```python
from build123d import *
from build123d.topology import SkipClean

# Parameters (mm, degrees)
EXTRUDE_1_DEPTH      = 2
SKETCH_3_W           = 2
SKETCH_3_H           = 2
EXTRUDE_3_DEPTH      = 4
SKETCH_4_W           = 1.3
SKETCH_4_H           = 2
EXTRUDE_4_DEPTH      = 6.5
SKETCH_5_W           = 2
SKETCH_5_H           = 11
EXTRUDE_5_DEPTH      = 2
CHAMFER_1_SIZE       = 0.5
SKETCH_6_R           = 1.5
CUT_EXTRUDE_1_DEPTH  = 2
EXTRUDE_6_DEPTH      = 2
EXTRUDE_6_DEPTH_BACK = 6
CUT_EXTRUDE_START    = -2
CUT_EXTRUDE_2_DEPTH  = 2


with BuildPart() as part:
    # 草图1 → 凸台-拉伸1 (new body)
    with BuildSketch(Plane(origin=(0, 0, 0), x_dir=(0, 0, -1), z_dir=(1, 0, 0))):
        Polygon((-5.5, -3), (5.5, -3), (5.5, 3), (3.4, 3), (3.4, 5), (1.4, 5), (1.4, 3), (-1.4, 3), (-1.4, 5), (-3.4, 5), (-3.4, 3), (-5.5, 3), align=None)
    extrude(amount=EXTRUDE_1_DEPTH)

    # 草图3 → 凸台-拉伸3 (add)
    with BuildSketch(Plane(origin=(2, 0, 0), x_dir=(0, 0, -1), z_dir=(1, 0, 0))):
        with Locations((-2.4, 4)):
            Rectangle(SKETCH_3_W, SKETCH_3_H)
        with Locations((2.4, 4)):
            Rectangle(SKETCH_3_W, SKETCH_3_H)
    extrude(amount=EXTRUDE_3_DEPTH)

    # 草图4 → 凸台-拉伸4 (add)
    with BuildSketch(Plane.XZ.offset(-3)):
        with Locations((5.35, 2.4)):
            Rectangle(SKETCH_4_W, SKETCH_4_H)
        with Locations((5.35, -2.4)):
            Rectangle(SKETCH_4_W, SKETCH_4_H)
    extrude(amount=EXTRUDE_4_DEPTH)

    # 草图5 → 凸台-拉伸5 (add)
    with BuildSketch(Plane.XZ.offset(3)):
        with Locations((1, 0)):
            Rectangle(SKETCH_5_W, SKETCH_5_H)
    extrude(amount=EXTRUDE_5_DEPTH)

    # 倒角1
    chamfer_1_edges = [part.edges().sort_by_distance(p)[0] for p in [
        (6, 5, -2.4),
        (6, 5, 2.4),
    ]]
    chamfer(chamfer_1_edges, length=CHAMFER_1_SIZE)

    # 草图6 → 切除-拉伸1 (cut)
    with BuildSketch(Plane.ZY):
        Circle(SKETCH_6_R)
    extrude(amount=-CUT_EXTRUDE_1_DEPTH, mode=Mode.SUBTRACT)

    # 草图2 → 凸台-拉伸6 (add, two sides: drawn at the far end of the back side and taken through both)
    with SkipClean():  # the faces are left unmerged after this step: merging them gives an invalid solid
        with BuildSketch(Plane.XZ.offset(3).offset(-EXTRUDE_6_DEPTH_BACK)):
            with BuildLine():
                Line((-2.3, 10.512451089), (-2.3, 9.464007706))
                ThreePointArc((-2.3, 9.464007706), (0.5, 0), (-2.3, -9.464007706))
                Line((-2.3, -9.464007706), (-2.3, -10.512451089))
                ThreePointArc((-2.3, -10.512451089), (-1.949751675, -10.989498714), (-1.389702257, -10.798205813))
                ThreePointArc((-1.389702257, -10.798205813), (2, 0), (-1.389702257, 10.798205813))
                ThreePointArc((-1.389702257, 10.798205813), (-1.949751675, 10.989498714), (-2.3, 10.512451089))
            make_face()
        extrude(amount=EXTRUDE_6_DEPTH + EXTRUDE_6_DEPTH_BACK)

    # 草图7 → 切除-拉伸2 (cut)
    with SkipClean():  # the faces are left unmerged after this step: merging them gives an invalid solid
        with BuildSketch(Plane(origin=(2, 0, 0), x_dir=(0, 0, -1), z_dir=(1, 0, 0)).offset(CUT_EXTRUDE_START)):
            with BuildLine():
                ThreePointArc((0, -1.5), (1.5, 0), (0, 1.5))
                ThreePointArc((0, 1.5), (-1.5, 0), (0, -1.5))
            make_face()
        extrude(amount=CUT_EXTRUDE_2_DEPTH, mode=Mode.SUBTRACT)


solid = part.part
```
Geometry: final body of the model. Coordinates: model frame, mm. A direction names the side the tool comes from. Coordinates: 2 decimals unless noted, no trailing zeros. Order: outer loops, then holes, each group sorted by start corner. A loop starts at its lowest first (then second) coordinate and runs counter-clockwise, first axis right, second up. Notation, with made-up numbers: (1.25, -18) -> (16.25, -18) arc R25 cw to (16.25, 4) -> close; hole circle Ø10 at (39.5, 61). An arc over 180 degrees is marked (long way). Answer in a Markdown table with one row per item.
Item 1: Section C-C on y = 2.25. Output: boundary loops of the cut face in (x, z).
Return value:
| item | result |
|---|---|
| outline | (-2.3, -10.51) arc R0.5 ccw to (-1.39, -10.8) arc R18.89 ccw to (1.18, -5.5) -> (2, -5.5) -> (2, 5.5) -> (1.18, 5.5) arc R18.89 ccw to (-1.39, 10.8) arc R0.5 ccw to (-2.3, 10.51) -> (-2.3, 9.46) arc R17.39 cw to (0, 4.14) -> (0, -4.14) arc R17.39 cw to (-2.3, -9.46) -> close; (4.7, -3.4) -> (6, -3.4) -> (6, -1.4) -> (4.7, -1.4) -> close; (4.7, 1.4) -> (6, 1.4) -> (6, 3.4) -> (4.7, 3.4) -> close |
Item 2: Contact query for flat-ended pins moving along their axis: P1, Ø0.6, axis at x = 2.5, z = -3, coming from the -Y side; P2, Ø2, axis at y = 2, z = 5.5, coming from the -X side; P3, Ø2, axis at x = 2, z = 7, coming from the -Y side; P4, Ø1.7, axis at x = 1.5, z = 0, coming from the +Y side. Output: stop coordinate, or through.
Return value:
| item | result |
|---|---|
| P1 | stops at y = 3 |
| P2 | stops at x = -0.76 |
| P3 | passes through |
| P4 | stops at y = 3 |
Item 3: Draft query along X for faces 5 (the cylindrical face through (0.086, -0.944, -8.287)), 6 (the flat face through (3, 3, -2)), 7 (the flat face through (-2.3, -1, -10)). Return one class per face: released by +X, released by -X, zero draft, split by the parting line, or undercut.
Return value:
| item | result |
|---|---|
| face 5 | released by +X |
| face 6 | undercut |
| face 7 | released by -X |
Item 4: Ray query, L1, parallel to Y at x = 0.45, z = 0; L2, parallel to X at y = 0.75, z = -2.5; L3, parallel to Z at x = 1.65, y = 0. Return the intervals inside material, ascending.
Return value:
| item | result |
|---|---|
| L1 | y = -5 to -1.5, 1.5 to 3 |
| L2 | x = 0 to 2, 4.7 to 6 |
| L3 | z = -5.5 to -1.5, 1.5 to 5.5 |
Item 5: Access query for faces 1 (the flat face through (5, 3, -3.4)), 2 (the cylindrical face through (-0.91, -0.94, -6.86)), 3 (the flat face through (4.7, 0, 2)), 4 (the flat face through (5, -3.5, 2)). Directions: +Z, -Z, +X, -X, +Y, -Y. A direction counts if a zero-diameter tool reaches every point of the face in a straight line with its end or side. Return the directions, or none.
Return value:
| item | result |
|---|---|
| face 1 | -Z, +X, +Y |
| face 2 | -X, +Y, -Y |
| face 3 | +Z, -Z, -Y |
| face 4 | +Z, -Z, +X, -Y |
Item 6: Section B-B on x = 4.25. Output: boundary loops of the cut face in (y, z).
Return value:
| item | result |
|---|---|
| outline | (3, -3.4) -> (5, -3.4) -> (5, -1.4) -> (3, -1.4) -> close; (3, 1.4) -> (5, 1.4) -> (5, 3.4) -> (3, 3.4) -> close |
Item 7: Section D-D on y = 0.75. Output: boundary loops of the cut face in (x, z), plus the area to 3 significant figures.
Return value:
| item | result |
|---|---|
| outline | (-2.3, -10.51) arc R0.5 ccw to (-1.39, -10.8) arc R18.89 ccw to (1.18, -5.5) -> (2, -5.5) -> (2, -1.3) -> (0, -1.3) -> (0, -4.14) arc R17.39 cw to (-2.3, -9.46) -> close; (-2.3, 9.46) arc R17.39 cw to (0, 4.14) -> (0, 1.3) -> (2, 1.3) -> (2, 5.5) -> (1.18, 5.5) arc R18.89 ccw to (-1.39, 10.8) arc R0.5 ccw to (-2.3, 10.51) -> close; (4.7, -3.4) -> (6, -3.4) -> (6, -1.4) -> (4.7, -1.4) -> close; (4.7, 1.4) -> (6, 1.4) -> (6, 3.4) -> (4.7, 3.4) -> close |
| area | 39.4 mm² |
Item 8: Section A-A on y = 3.75. Output: boundary loops of the cut face in (x, z).
Return value:
| item | result |
|---|---|
| outline | (0, -3.4) -> (6, -3.4) -> (6, -1.4) -> (0, -1.4) -> close; (0, 1.4) -> (6, 1.4) -> (6, 3.4) -> (0, 3.4) -> close |
